Can you work these out from the drawing? Everything is in mm from the part's minimum corner. Coordinates: 2 decimals unless noted, no trailing zeros. Loops run counter-clockwise (first coordinate to the right, second up) from the corner with the lowest first, then second, coordinate; pieces in that order, holes last. Notation, with made-up numbers: (27, -36.75) -> (71, -36.75) arc R14 ccw to (71, -10.75) -> close; hole circle Ø6 at (36, -19.75). An arc over 180 degrees is marked (long way). One line per question, with ' | ' between items.
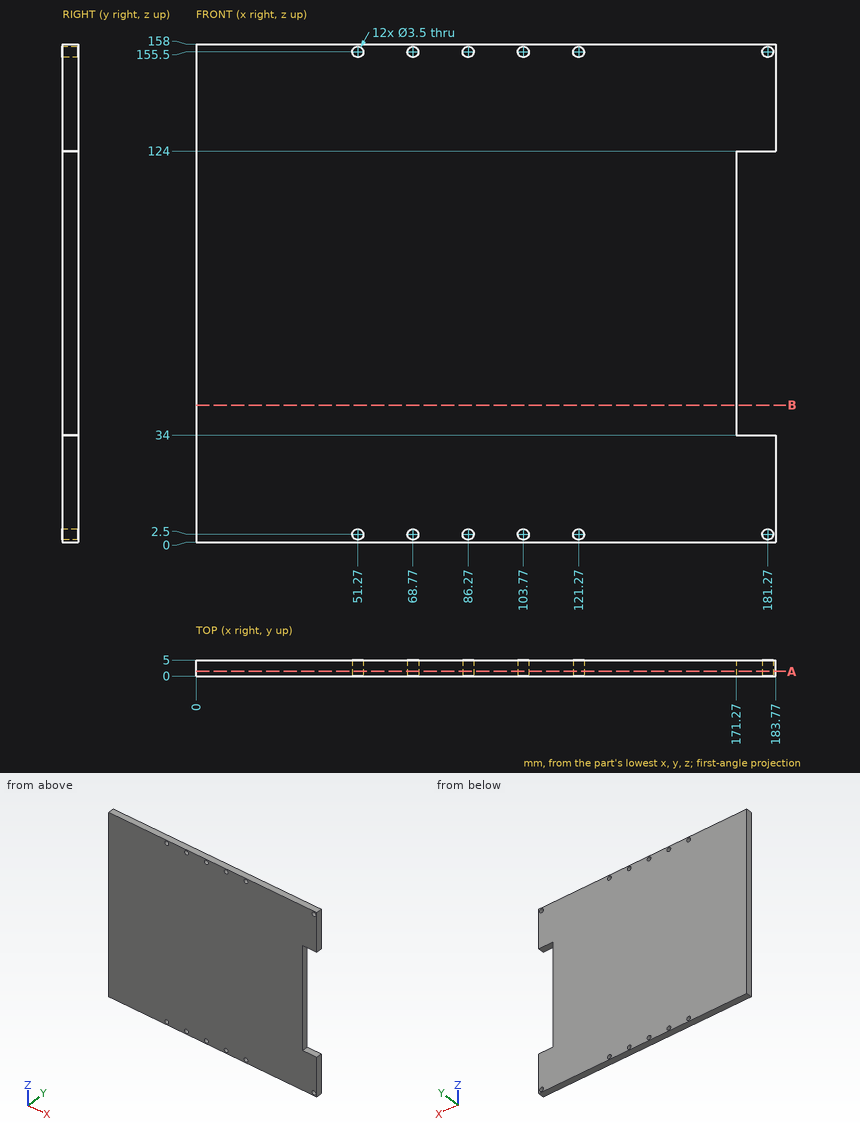
Q1. Please list where these lines run through material, in increasing order: L1, parallel to Z at x = 51.27, y = 2.65; L2, parallel to X at y = 4.55, z = 85.5. Write a range as [from, to].
Values follow:
L1: z = [0, 0.75], [4.25, 153.75], [157.25, 158] | L2: x = [0, 171.27]
Q2. Imagine slicing it at B-B on z = 43.5. Write out the boundary of the cut face in (x, y).
Values follow:
outline: (0, 0) -> (171.27, 0) -> (171.27, 5) -> (0, 5) -> close
Q3. Imagine slicing it at A-A on y = 1.5. Give the number of separate pieces and of enclosed holes in the cut face, plus the area to 3 significant figures.
Values follow:
separate pieces: 1 | enclosed holes: 12 | area: 27,800 mm2
Q4. For pin 1 (5.5 mm diameter, centred on x = 86.27, z = 155.5, fed in from -Y); pin 2 (2.5 mm diameter, centred on y = 2.5, z = 100, fed in from +X), each with a flat end and sliding along its axis, tell me the tip position at first contact or that it passes through.
Values follow:
pin 1: stops at y = 0 | pin 2: stops at x = 171.27
